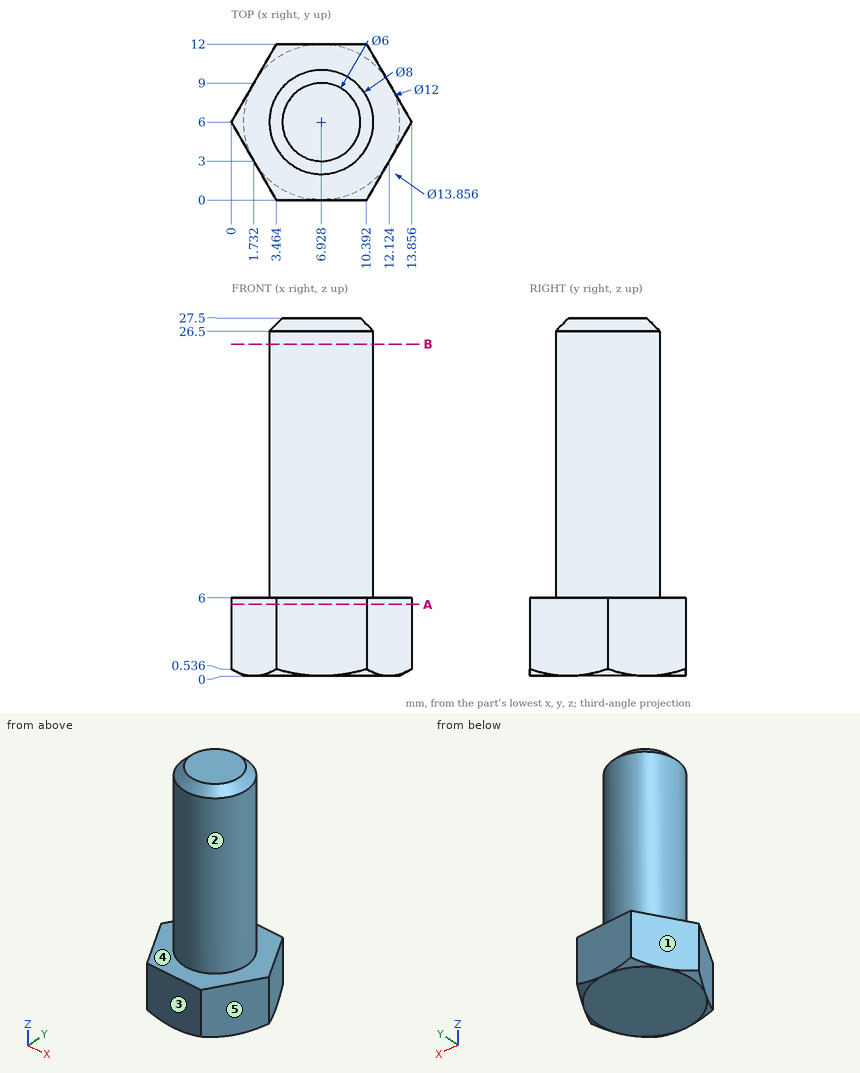
Input: dimensioned drawing with shaded views. Units: mm. Origin: part minimum x, y, z. A direction names the side the tool comes from. Give positions to 0.01 mm unless a question says otherwise; leave off trailing zeros. Loops run counter-clockwise (first coordinate to the right, second up) from the corner with the lowest first, then second, coordinate; pieces in that order, holes last. Notation, with made-up numbers: (-4, -26.75) -> (48, -26.75) arc R9 cw to (48, -14.75) -> close; hole circle Ø6 at (-9, -29). An arc over 180 degrees is marked (long way). Use a Markdown table: item, result. Add a question column.
1) Section query A-A, the plane z = 5.5. Return the cut outline in (x, y), then the cut area to 3 significant figures.
2) Reachability of the marked faces 4 and 5 from +Z, -Z, +X, -X, +Y, -Y: full face, straight path, thin tool, end or side. Return the list, or none.
3) Line query: line 1 along Z through (x, y) = (2.75, 6.25); line 2 along X through (y, z) = (4.5, 18.25) (1 decimal); line 3 along Z through (x, y) = (3, 11). Output: solid intervals per line, ascending. Write a range as [from, to].
4) Section query B-B, the plane z = 25.5. Return the cut outline in (x, y).
5) First-contact query: pin 1 (4 mm diameter, centred on x = 10.5, z = 16.5, fed in from -Y); pin 2 (1.5 mm diameter, centred on x = 6.5, z = 10.5, fed in from +Y); pin 3 (5 mm diameter, centred on y = 9, z = 14.5, fed in from -X). Flat tips, straight axial feed; report the tip coordinate or a pass-through.
6) Pull-direction query (X, two-part tool) for the marked faces 1, 2 and 3; classes: +X half, -X half, draft (parallel to the pull), parting line (faces both ways), or undercut.
Numbers:
| question | item | result |
|---|---|---|
| 1 | outline | (0, 6) -> (3.46, 0) -> (10.39, 0) -> (13.86, 6) -> (10.39, 12) -> (3.46, 12) -> close |
| 1 | area | 125 mm2 |
| 2 | face 4 | +Z |
| 2 | face 5 | +Z, -Z, +X, -Y |
| 3 | line 1 | z = [0, 6] |
| 3 | line 2 | x = [3.2, 10.6] |
| 3 | line 3 | z = [0.21, 6] |
| 4 | outline | circle Ø8 at (6.93, 6) |
| 5 | pin 1 | stops at y = 2.32 |
| 5 | pin 2 | stops at y = 10 |
| 5 | pin 3 | stops at x = 2.96 |
| 6 | face 1 | -X half |
| 6 | face 2 | parting line |
| 6 | face 3 | draft |
